Autodesk Inventor part; units mm, degrees
ref_plane "YZ Plane" through (0, 0, 0) normal (1, 0, 0) x (0, 1, 0)
ref_plane "XZ Plane" through (0, 0, 0) normal (0, 1, 0) x (-1, 0, 0)
ref_plane "XY Plane" through (0, 0, 0) normal (0, 0, 1) x (1, 0, 0)
sketch "Sketch1" plane through (0, 0, 0) normal (0, 0, 1) x (1, 0, 0)
  line L0 (0, 0) -> (9.525, 0)
  line L1 (88.9, 0) -> (88.9, 63.5)
  line L2 (88.9, 63.5) -> (0, 63.5)
  line L3 (0, 63.5) -> (0, 0)
  line L4 (79.375, 0) -> (79.375, -12.7)
  line L5 (79.375, -12.7) -> (73.025, -12.7)
  line L6 (73.025, -12.7) -> (73.025, 0)
  line L7 (44.45, 0) -> (44.45, 63.5) construction
  line L8 (16.25, 0) -> (16.25, 56.4) construction
  line L9 (16.25, 56.4) -> (72.65, 56.4) construction
  line L10 (72.65, 56.4) -> (72.65, 0) construction
  line L11 (9.525, 0) -> (9.525, -12.7)
  line L12 (9.525, -12.7) -> (15.875, -12.7)
  line L13 (15.875, -12.7) -> (15.875, 0)
  line L14 (15.875, 0) -> (73.025, 0)
  line L15 (79.375, 0) -> (88.9, 0)
  dimension "d0" = 88.9
  dimension "d1" = 63.5
  dimension "d4" = 6.35
  dimension "d5" = 12.7
ref_plane "Work Plane1" through (0, 0, 12.7) normal (0, 0, 1) x (1, 0, 0)
sketch "Sketch2" plane through (0, 0, 12.7) normal (0, 0, 1) x (1, 0, 0)
  line L0 (23.3366, 59.575) -> (23.3366, 49.3134)
  line L1 (65.5634, 51.3062) -> (65.5634, 49.3134)
  line L2 (65.5634, 59.575) -> (65.5634, 49.3134)
  line L3 (23.3366, 49.3134) -> (23.3366, 56.4)
  line L4 (65.5634, 49.3134) -> (72.65, 49.3134)
  line L5 (72.65, 49.3134) -> (72.65, 7.0866)
  line L6 (72.65, 7.0866) -> (65.5634, 7.0866)
  line L7 (23.3366, 7.0866) -> (23.3366, 0)
  line L8 (23.3366, 0) -> (65.5634, 0)
  line L9 (65.5634, 0) -> (65.5634, 7.0866)
  line L10 (23.3366, 7.0866) -> (16.25, 7.0866)
  line L11 (16.25, 7.0866) -> (16.25, 49.3134)
  line L12 (16.25, 49.3134) -> (23.3366, 49.3134)
  line L13 (44.45, 0) -> (44.45, 56.4) construction
  line L14 (28.575, 0) -> (60.325, 0) construction
  line L15 (44.45, 0) -> (44.45, 63.5) construction
  line L16 (88.9, 63.5) -> (0, 63.5) construction
  line L17 (72.65, 0) -> (16.25, 0) construction
  line L18 (16.25, 0) -> (16.25, 56.4) construction
  line L19 (72.65, 56.4) -> (72.65, 0) construction
  line L20 (23.3366, 59.575) -> (65.5634, 59.575)
  point P0 (0, 0)
  point P1 (72.65, 56.4)
extrude "Extrusion3" add sketch "Sketch1" along normal blind 12.7
extrude "Extrusion5" cut sketch "Sketch2" against normal blind 8.763
sketch "Sketch3" plane through (0, 0, 12.7) normal (0, 0, 1) x (1, 0, 0)
  line L0 (0, 63.5) -> (0, 0) construction
  line L1 (0, 63.5) -> (0, 0) construction
  line L2 (0, 25.4) -> (6.35, 25.4)
  line L3 (6.35, 25.4) -> (6.35, 38.1)
  line L4 (6.35, 38.1) -> (0, 38.1)
  line L5 (0, 38.1) -> (0, 25.4)
  line L6 (88.9, 63.5) -> (0, 63.5) construction
  line L7 (44.45, 63.5) -> (44.45, 0) construction
  line L8 (65.5634, 0) -> (23.3366, 0) construction
  line L9 (88.9, 25.4) -> (82.55, 25.4)
  line L10 (82.55, 25.4) -> (82.55, 38.1)
  line L11 (82.55, 38.1) -> (88.9, 38.1)
  line L12 (88.9, 38.1) -> (88.9, 25.4)
  point P0 (0, 31.75)
  point P1 (88.9, 31.75)
  dimension "d19" = 12.7
extrude "Extrusion6" cut sketch "Sketch3" against normal through all
sketch "Sketch4" plane through (0, 0, 12.7) normal (0, 0, 1) x (1, 0, 0)
  line L0 (88.9, 63.5) -> (0, 63.5) construction
  line L1 (44.45, 63.5) -> (44.45, 69.85) construction
  line L2 (44.45, 63.5) -> (50.8, 63.5) construction
  line L3 (38.1, 63.5) -> (50.8, 63.5)
  line L4 (50.8, 63.5) -> (50.8, 76.2)
  line L5 (50.8, 76.2) -> (38.1, 76.2)
  line L6 (38.1, 76.2) -> (38.1, 63.5)
  line L7 (38.1, 63.5) -> (50.8, 76.2) construction
  line L8 (50.8, 63.5) -> (38.1, 76.2) construction
  point P0 (0, 0)
  dimension "d22" = 6.35
  dimension "d23" = 90
  dimension "d24" = 12.7
  dimension "d25" = 12.7
extrude "Extrusion7" add sketch "Sketch4" against normal blind 12.7
fillet "Fillet1" radius 6.35 1 edges at (44.45, 76.2, 0)
properties part number "Near End Cap" material "PVC-Piping"
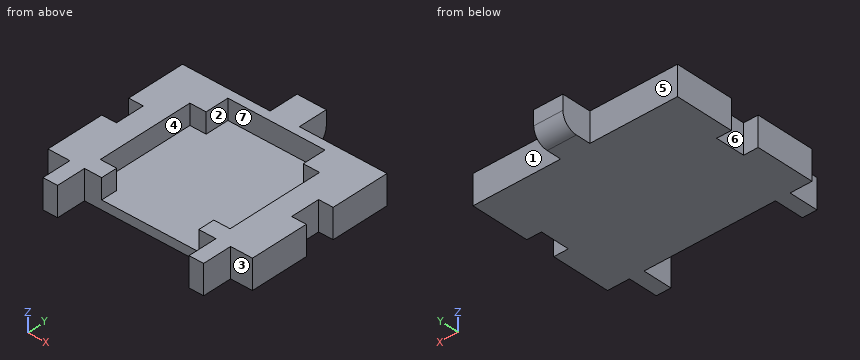
Model file for the job. Use its own axes, mm. Face numbers are marked on the shaded views. A direction names the side the tool comes from. Coordinates: 2 decimals unless noted, no trailing zeros. Order: outer loops, then holes, each group sorted by start corner. A loop starts at its lowest first (then second) coordinate and runs counter-clockwise, first axis right, second up. Notation, with made-up numbers: M 26,44 L 83,44 A18 cw 83,78 Z; hole C -5.75,75 d7. An arc over 180 degrees is marked long. Return JSON: item names as keys, results as strings.
1. Saw through at D-D (y = 2). Give the cut face in (x, z).
Ans:
{"outline": "M 0,0 L 88.9,0 L 88.9,12.7 L 65.56,12.7 L 65.56,3.94 L 23.34,3.94 L 23.34,12.7 L 0,12.7 Z"}
2. Saw through at A-A (x = 49). Give the cut face in (y, z) (3 decimals).
Ans:
{"outline": "M 0,0 L 69.85,0 A6.35 ccw 76.2,6.35 L 76.2,12.7 L 59.575,12.7 L 59.575,3.937 L 0,3.937 Z"}
3. Drill centre lines: probe 1 along X at (y, z) = (55, 10.25); probe 2 along X at (y, z) = (-0.5, 5.5) (3 decimals); probe 3 along Y at (x, z) = (68, 8.5). Where is each one in solid material? Low to high.
Ans:
{"probe 1": "0 to 23.34, 65.56 to 88.9", "probe 2": "9.525 to 15.875, 73.025 to 79.375", "probe 3": "0 to 7.09, 49.31 to 63.5"}
4. Saw through at B-B (y = 20). Give the cut face in (x, z), and give its area (3 significant figures).
Ans:
{"outline": "M 0,0 L 88.9,0 L 88.9,12.7 L 72.65,12.7 L 72.65,3.94 L 16.25,3.94 L 16.25,12.7 L 0,12.7 Z", "area": "635 mm^2"}
5. Flat gauge pins, fed straight in: pin 1 (4.5 mm diameter, centred on y = 28, z = 9, fed in from +X); pin 2 (5.5 mm diameter, centred on x = 68, z = 10.5, fed in from -Y); pin 3 (6.5 mm diameter, centred on x = 12.5, z = 8, fed in from +Y). Where does each tip first touch, or does it go through?
Ans:
{"pin 1": "x = 82.55", "pin 2": "y = 0", "pin 3": "y = 63.5"}
6. Saw through at C-C (z = 2.75). Give the cut face in (x, y) (3 decimals).
Ans:
{"outline": "M 0,0 L 9.525,0 L 9.525,-12.7 L 15.875,-12.7 L 15.875,0 L 73.025,0 L 73.025,-12.7 L 79.375,-12.7 L 79.375,0 L 88.9,0 L 88.9,25.4 L 82.55,25.4 L 82.55,38.1 L 88.9,38.1 L 88.9,63.5 L 50.8,63.5 L 50.8,75.081 L 38.1,75.081 L 38.1,63.5 L 0,63.5 L 0,38.1 L 6.35,38.1 L 6.35,25.4 L 0,25.4 Z"}
7. Tool access for the marked faces 1, 2 and 3: list every direction of +Z, -Z, +X, -X, +Y, -Y with a clear straight run to the whole face (end or side of a thin tool).
Ans:
{"face 1": "+Z, -Z, +X, +Y", "face 2": "+Z, -Y", "face 3": "+Z, -Z, +X, -Y"}
8. Pull direction Y, two halves, no side cores. Call the marked faces 4, 5, 6 and 7: +Y half, -Y half, draft (parallel to the pull), parting line (faces both ways), or undercut.
Ans:
{"face 4": "undercut", "face 5": "+Y half", "face 6": "undercut", "face 7": "-Y half"}
